Part model, mm, in its own coordinate system. Face numbers are marked on the shaded views. A direction names the side the tool comes from. Give positions to 0.01 mm unless a question says otherwise; leave off trailing zeros. Write each loop counter-clockwise with the first axis right and the second up, starting at its lowest first coordinate (ties: lowest second). Pieces come first, ordered by that corner, then holes. Notation, with made-up numbers: M 36.25,-15.75 L 81.25,-15.75 A33 cw 81.25,16.25 Z; hole C 61,69.5 d9. An arc over 180 degrees is marked long. Use a Markdown table: item, result. Add a question column.
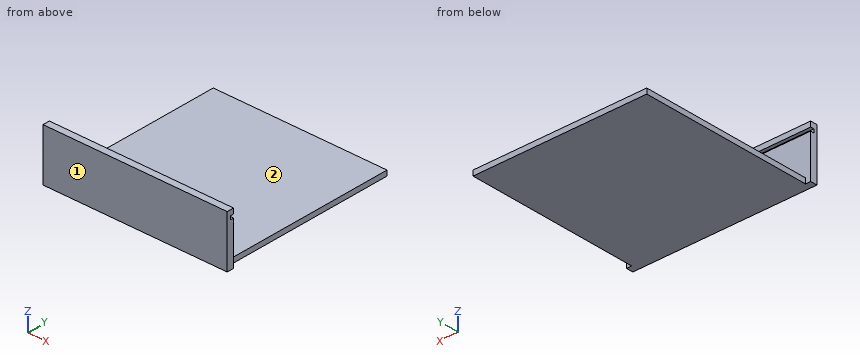
from build123d import *

# Parameters (mm, degrees)
F0_W     = 100
F0_H     = 100
F1_DEPTH = 3
F2_W     = 106
F2_H     = 25
F2_H_2   = 2
F2_H_3   = 3
F3_DEPTH = 4
F4_W     = 106
F4_H     = 2
F5_DEPTH = 2


with BuildPart() as f1:
    # F0 (on Top) → F1 (new body)
    with BuildSketch(Plane.XY):
        Rectangle(F0_W, F0_H)
    extrude(amount=-F1_DEPTH)

    # F2 (on face) → F3 (join)
    with BuildSketch(Plane.XZ.offset(50)):
        with Locations((0, 9.5)):
            Rectangle(F2_W, F2_H)
        with Locations((0, 23)):
            Rectangle(F2_W, F2_H_2)
        with Locations((0, 25.5)):
            Rectangle(F2_W, F2_H_3)
    extrude(amount=F3_DEPTH)

    # F4 (on face) → F5 (cut)
    with BuildSketch(Plane(origin=(0, -50, 0), x_dir=(-1, 0, 0), z_dir=(0, 1, 0))):
        with Locations((0, 23)):
            Rectangle(F4_W, F4_H)
    extrude(amount=-F5_DEPTH, mode=Mode.SUBTRACT)


solid = f1.part
1. Drill centre lines: probe 1 along Z at (x, y) = (4, 10); probe 2 along Y at (x, z) = (-5.5, 23.75); probe 3 along Y at (x, z) = (-38.5, 0.5). Where is each one in solid material? Low to high. Write a range as [from, to].
2. Tool access for the marked faces 1 and 2: list every direction of +Z, -Z, +X, -X, +Y, -Y with a clear straight run to the whole face (end or side of a thin tool).
3. Flat gauge pins, fed straight in: pin 1 (5 mm diameter, centred on x = -16, z = 5, fed in from +Y); pin 2 (1.5 mm diameter, centred on y = 2, z = -2, fed in from -X); pin 3 (2.5 mm diameter, centred on y = -7.5, z = -1, fed in from +X). Where does each tip first touch, or does it go through?
4. Cut at B-B (y = -15.5). Write the cut outline in (x, z).
5. Cut at A-A (x = 40). Write the cut outline in (y, z).
6. Cut at C-C (z = 19). Write the cut outline in (x, y), then the cut area to 3 significant figures.
A:
| question | item | result |
|---|---|---|
| 1 | probe 1 | z = [-3, 0] |
| 1 | probe 2 | y = [-54, -52] |
| 1 | probe 3 | y = [-54, -50] |
| 2 | face 1 | +Z, -Z, +X, -X, -Y |
| 2 | face 2 | +Z, +X, -X, +Y |
| 3 | pin 1 | stops at y = -50 |
| 3 | pin 2 | stops at x = -50 |
| 3 | pin 3 | stops at x = 50 |
| 4 | outline | M -50,-3 L 50,-3 L 50,0 L -50,0 Z |
| 5 | outline | M -54,-3 L 50,-3 L 50,0 L -50,0 L -50,22 L -52,22 L -52,24 L -50,24 L -50,27 L -54,27 Z |
| 6 | outline | M -53,-54 L 53,-54 L 53,-50 L -53,-50 Z |
| 6 | area | 424 mm² |
